```python
from build123d import *

# Parameters (mm, degrees)
SKETCH1_R           = 3
SKETCH1_R_2         = 1.65
BOSS_EXTRUDE1_DEPTH = 9
BOSS_EXTRUDE2_DEPTH = 5
BOSS_EXTRUDE3_START = -3
SKETCH2_3_R         = 3
BOSS_EXTRUDE3_DEPTH = 3
FILLET1_R           = 4
FILLET2_R           = 0.5


with BuildPart() as part:
    # Sketch1 → Boss-Extrude1 (new body)
    with BuildSketch(Plane(origin=(0, 0, 0), x_dir=(1, 0, 0), z_dir=(0, 1, 0))):
        with Locations(Location((0, 0, 0), (0, 0, 270))):
            Circle(SKETCH1_R)
        with Locations(Location((0, 0, 0), (0, 0, 270))):
            Circle(SKETCH1_R_2, mode=Mode.SUBTRACT)
    extrude(amount=BOSS_EXTRUDE1_DEPTH)



with BuildPart() as body_2:
    # Sketch2 → Boss-Extrude2 (new body)
    with BuildSketch(Plane(origin=(0, 9, 0), x_dir=(1, 0, 0), z_dir=(0, 1, 0))):
        Polygon((-0.41717713, 8.014318223), (-7.14919174, 3.645873119), (-6.73201461, -4.368445104), (0.41717713, -8.014318223), (7.14919174, -3.645873119), (6.73201461, 4.368445104), align=None)
        Polygon((-4.794744219, -3.111338599), (0.297126157, -5.708039598), (5.091870376, -2.596700998), (4.794744219, 3.111338599), (-0.297126157, 5.708039598), (-5.091870376, 2.596700998), align=None, mode=Mode.SUBTRACT)
    extrude(amount=BOSS_EXTRUDE2_DEPTH)


with BuildPart() as part_1:
    add(part.part)

    add(body_2.part)  # Boss-Extrude3 merges body 2
    # Sketch2_3 → Boss-Extrude3 (add)
    # profile 1 of 2: a face of its own
    with BuildSketch(Plane(origin=(0, 9, 0), x_dir=(1, 0, 0), z_dir=(0, 1, 0)).offset(BOSS_EXTRUDE3_START)):
        Polygon((7.14919174, -3.645873119), (6.73201461, 4.368445104), (-0.41717713, 8.014318223), (-7.14919174, 3.645873119), (-6.73201461, -4.368445104), (0.41717713, -8.014318223), align=None)
        Polygon((-5.091870376, 2.596700998), (-4.794744219, -3.111338599), (0.297126157, -5.708039598), (5.091870376, -2.596700998), (4.794744219, 3.111338599), (-0.297126157, 5.708039598), align=None, mode=Mode.SUBTRACT)
    # profile 2 of 2: a face of its own
    with BuildSketch(Plane(origin=(0, 9, 0), x_dir=(1, 0, 0), z_dir=(0, 1, 0)).offset(BOSS_EXTRUDE3_START)):
        Polygon((-0.297126157, 5.708039598), (-5.091870376, 2.596700998), (-4.794744219, -3.111338599), (0.297126157, -5.708039598), (5.091870376, -2.596700998), (4.794744219, 3.111338599), align=None)
        with Locations(Location((0, 0, 0), (0, 0, 270))):
            Circle(SKETCH2_3_R, mode=Mode.SUBTRACT)
    extrude(amount=BOSS_EXTRUDE3_DEPTH)

    # Fillet1
    # the kernel refuses this fillet: 4 mm, written as the material it adds along each edge
    with BuildSketch(Plane(origin=(0, 6, 0), x_dir=(0, 0, 1), z_dir=(-1, 0, 0))) as fillet1_piece_1_section:
        with BuildLine():
            CenterArc((3 + FILLET1_R, -FILLET1_R), FILLET1_R, 90, 90)
            Line((3 + FILLET1_R, 0), (3, 0))
            Line((3, 0), (3, -FILLET1_R))
        make_face()
    fillet1_piece_1 = revolve(axis=Axis((0, 6, 0), (0, 1, 0)), mode=Mode.PRIVATE)
    fillet1_piece_1 = split(fillet1_piece_1, bisect_by=Plane(origin=(6.725747401, 4.861258517, -4.488843378), z_dir=(-0.998647938837555, 0, 0.05198359602319992)), keep=Keep.TOP, mode=Mode.PRIVATE)
    fillet1_piece_1 = split(fillet1_piece_1, bisect_by=Plane(origin=(1.482404707, 4.861258517, -7.045588524), z_dir=(-0.4543048546826189, 0, 0.8908462824818909)), keep=Keep.TOP, mode=Mode.PRIVATE)
    fillet1_piece_1 = split(fillet1_piece_1, bisect_by=Plane(origin=(-1.893314628, 4.861258517, -7.056443649), z_dir=(0.544343084154936, 0, 0.8388626864586911)), keep=Keep.TOP, mode=Mode.PRIVATE)
    fillet1_piece_1 = split(fillet1_piece_1, bisect_by=Plane(origin=(-7.155458949, 4.861258517, -3.766271394), z_dir=(0.998647938837555, 0, -0.051983596023199824)), keep=Keep.TOP, mode=Mode.PRIVATE)
    fillet1_piece_1 = split(fillet1_piece_1, bisect_by=Plane(origin=(-4.832432773, 4.861258517, 5.337174802), z_dir=(0.4543048546826189, 0, -0.8908462824818907)), keep=Keep.TOP, mode=Mode.PRIVATE)
    fillet1_piece_1 = split(fillet1_piece_1, bisect_by=Plane(origin=(5.673054242, 4.861258517, 4.603747693), z_dir=(-0.5443430841549362, 0, -0.8388626864586911)), keep=Keep.TOP, mode=Mode.PRIVATE)
    add(fillet1_piece_1)

    # Fillet2
    fillet2_edges = [part_1.edges().sort_by_distance(p)[0] for p in [
        (-4.943307297, 14, 0.2573188),
        (-2.248809031, 14, 4.409689098),
        (2.694498267, 14, 4.152370298),
        (4.943307297, 14, -0.2573188),
        (2.248809031, 14, -4.409689098),
        (-2.694498267, 14, -4.152370298),
    ]]
    fillet(fillet2_edges, radius=FILLET2_R)


solid = part_1.part
```
Design review of the part built by this model. Coordinates are the model's own, in mm. A direction names the side the tool comes from. Give positions to 0.01 mm unless a question says otherwise; leave off trailing zeros. Loops run counter-clockwise (first coordinate to the right, second up) from the corner with the lowest first, then second, coordinate; pieces in that order, holes last. Notation, with made-up numbers: M 76,39.25 L 91,39.25 A31 cw 91,74.25 Z; hole C 31.5,37 d6. An arc over 180 degrees is marked long. Return JSON: item names as keys, results as strings. Group by question number.
Item 1: Tool access review of faces 5 (the flat face through (6, 6, -4)), 6 (the cylindrical face through (-2.813, 13.857, -4.255)), 7 (the flat face through (-6, 6, 4)): name each direction out of +Z, -Z, +X, -X, +Y, -Y from which nothing blocks a thin tool from reaching the whole face with its end or side.
Item 2: We need section B-B (y = 2.75). Give the boundary of the cut face in (x, z).
Item 3: Mouldability with a two-part tool opening along Z and no side actions: class faces 1 (the cylindrical face through (2.278, 13.857, -4.564)), 2 (the flat face through (6.4, 6, 3.3)), 3 (the cylindrical face through (-2.278, 13.857, 4.564)), 4 (the cylindrical face through (0.9, 0.99, 2.86)) as released by +Z, released by -Z, zero draft, split by the parting line, or undercut.
Item 4: For probe 1 along X at (y, z) = (2.5, 0); probe 2 along X at (y, z) = (12.5, -5.25); probe 3 along Y at (x, z) = (-1.5, -3), list the stretches that pass through material, from the lowest coordinate up.
Item 5: We need section A-A (y = 10). Give the boundary of the cut face in (x, z).
Item 6: Insertion check: pin 1 Ø8 at (x, y) = (-5, 7.5) entering from +Z; pin 2 Ø1.9 at (x, z) = (0, 7.5) entering from -Y; pin 3 Ø2 at (x, z) = (-2.5, 3.5) entering from -Y. Each pin has a flat end and moves straight along its axis. Give the tip position at first contact, or say it passes through.
Output:
{
 "1": {"face 5": "-Z, +X, -Y", "face 6": "+Y", "face 7": "+Z, -X, -Y"},
 "2": {"outline": "C 0,0 d6.14; hole C 0,0 d3.3"},
 "3": {"face 1": "undercut", "face 2": "zero draft", "face 3": "undercut", "face 4": "split by the parting line"},
 "4": {"probe 1": "x = -3.03 to -1.65, 1.65 to 3.03", "probe 2": "x = -4.68 to -1, 0.6 to 5", "probe 3": "y = 3.65 to 9"},
 "5": {"outline": "M -7.15,-3.65 L -0.42,-8.01 L 6.73,-4.37 L 7.15,3.65 L 0.42,8.01 L -6.73,4.37 Z; hole M -5.09,-2.6 L -0.3,-5.71 L 4.79,-3.11 L 5.09,2.6 L 0.3,5.71 L -4.79,3.11 Z"},
 "6": {"pin 1": "stops at z = 7.29", "pin 2": "stops at y = 5.97", "pin 3": "stops at y = 3.52"}
}
